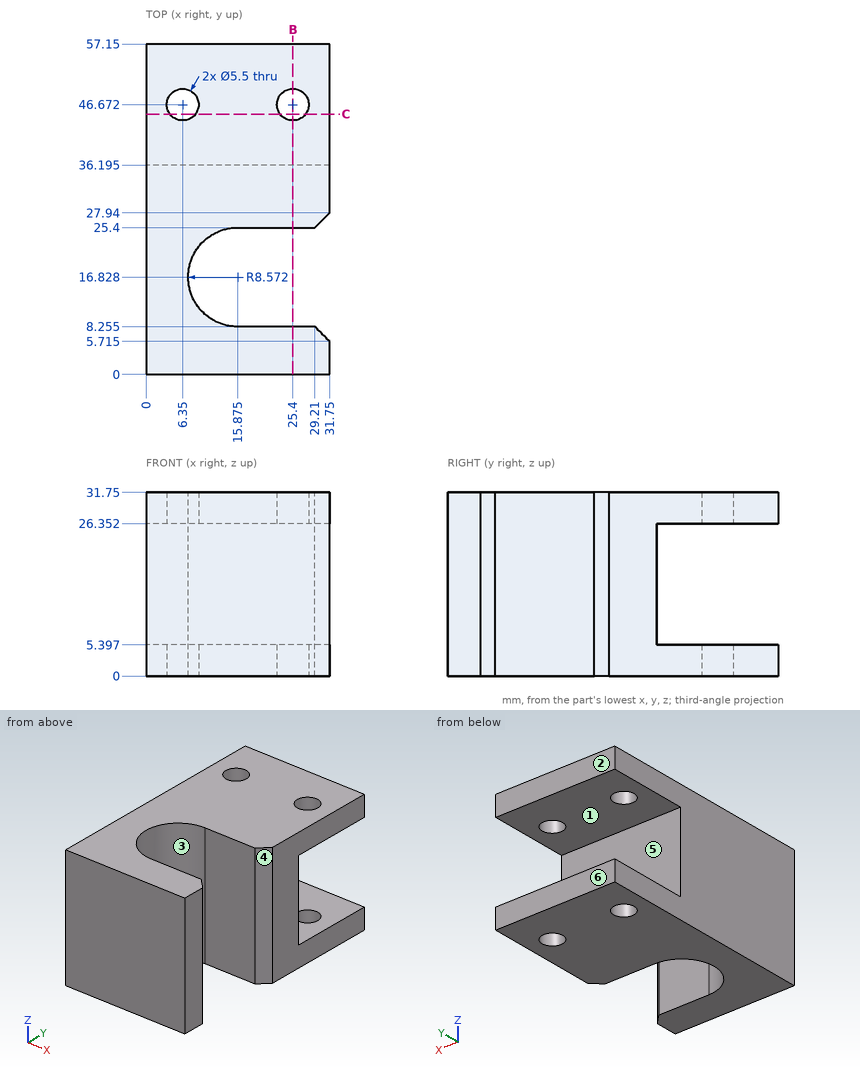
Verification items for this drawing (mm, ordinates from the low corner). A direction names the side the tool comes from. Coordinates: 2 decimals unless noted, no trailing zeros. Write each loop counter-clockwise with the first axis right and the second up, starting at its lowest first coordinate (ties: lowest second). Pieces come first, ordered by that corner, then holes. Notation, with made-up numbers: M -23,11.5 L 33,11.5 A30 cw 33,46.5 Z; hole C 26,-21 d5. An arc over 180 degrees is marked long. Answer as a JSON object with one key per item and string values. Group by question number.
(1) Cross-section at C-C, the plane y = 45. Record the cut outline in (x, z).
(2) Gauge pin test, flat ends, axial feed: pin 1 (7 mm diameter, centred on x = 6.35, y = 46.67, fed in from +Z); pin 2 (6.5 mm diameter, centred on x = 14.5, z = 13.5, fed in from +Y) (1 decimal). Record the tip position at first contact, or that the pin passes through.
(3) Tool access check on the marked faces 4, 5 and 6. Record the directions out of +Z, -Z, +X, -X, +Y, -Y that give a thin tool (end or side, any length) a straight path to the whole face; none if there is none.
(4) Release check for a two-part mould opening along Y. For the marked faces 1, 2 and 3 record: +Y half, -Y half, draft (parallel to the pull), parting line (faces both ways), or undercut.
(5) Cross-section at B-B, the plane x = 25.4. State how many separate pieces and enclosed holes the cut face has.
(6) Material ranges on line 1 (Y direction, x = 6.35, z = 3.6); line 2 (Z direction, x = 18, y = 50.5); line 3 (Y direction, x = 28.5, z = 17.5) (1 decimal), recorded low to high.
Reply:
{
 "1": {"outline": "M 0,0 L 4.17,0 L 4.17,5.4 L 0,5.4 Z; M 0,26.35 L 4.17,26.35 L 4.17,31.75 L 0,31.75 Z; M 8.53,0 L 23.22,0 L 23.22,5.4 L 8.53,5.4 Z; M 8.53,26.35 L 23.22,26.35 L 23.22,31.75 L 8.53,31.75 Z; M 27.58,0 L 31.75,0 L 31.75,5.4 L 27.58,5.4 Z; M 27.58,26.35 L 31.75,26.35 L 31.75,31.75 L 27.58,31.75 Z"},
 "2": {"pin 1": "z = 31.75", "pin 2": "y = 36.2"},
 "3": {"face 4": "+Z, -Z, +X", "face 5": "+X, -X, +Y", "face 6": "+Z, -Z, +X, -X, +Y"},
 "4": {"face 1": "draft", "face 2": "+Y half", "face 3": "undercut"},
 "5": {"separate pieces": "4", "enclosed holes": "0"},
 "6": {"line 1": "0 to 43.92, 49.42 to 57.15", "line 2": "0 to 5.4, 26.35 to 31.75", "line 3": "0 to 8.3, 25.4 to 36.2"}
}
